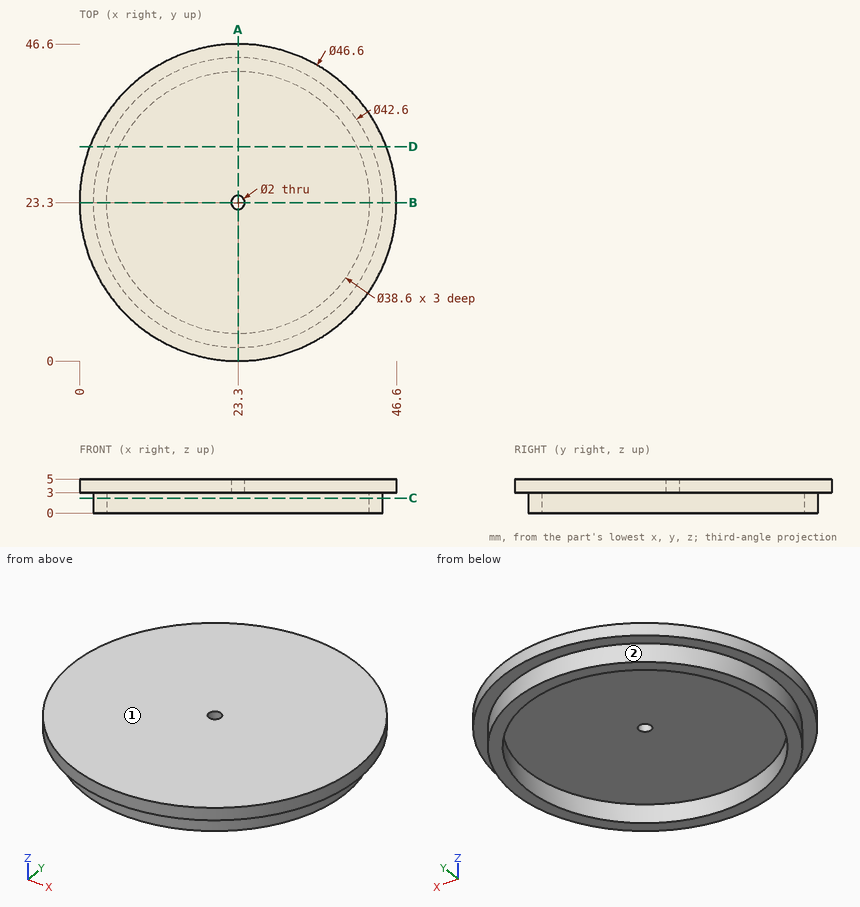
Print and shaded views of the part. All mm, measured from the part's lowest x, y and z. A direction names the side the tool comes from. Coordinates: 2 decimals unless noted, no trailing zeros. Order: outer loops, then holes, each group sorted by start corner. A loop starts at its lowest first (then second) coordinate and runs counter-clockwise, first axis right, second up. Notation, with made-up numbers: (49, -12) -> (64, -12) arc R11 cw to (64, -8) -> close; hole circle Ø6 at (30.25, 66). An arc over 180 degrees is marked (long way). Use one line per item in the form item = value. Start each with the question number.
1) Band-saw the part on C-C on z = 2.2. Give the cut face in (x, y), then the cut area to 3 significant figures.
2) Drill centre lines: L1, parallel to Y at x = 23, z = 2.5; L2, parallel to Y at x = 23.3, z = 3.4; L3, parallel to Z at x = 32, y = 44. Where is each one in solid material? Low to high. Write a range as [from, to].
3) Band-saw the part on D-D on y = 31.5. Give the cut face in (x, z).
4) Band-saw the part on A-A on x = 23.3. Give the cut face in (y, z).
5) Tool access for the marked faces 1 and 2: list every direction of +Z, -Z, +X, -X, +Y, -Y with a clear straight run to the whole face (end or side of a thin tool).
6) Drop flat-ended pins along their axis: pin 1 (3 mm diameter, centred on y = 10, z = 3, fed in from -X); pin 2 (3 mm diameter, centred on y = 16.5, z = 2, fed in from +X); pin 3 (1.5 mm diameter, centred on y = 31, z = 1, fed in from +X); pin 4 (1.2 mm diameter, centred on x = 23.3, y = 23.3, fed in from +Z). Give the stop position or say it passes through.
Entries:
q1.outline = circle Ø42.6 at (23.3, 23.3); hole circle Ø38.6 at (23.3, 23.3)
q1.area = 255 mm2
q2.L1 = [2, 4], [42.6, 44.6]
q2.L2 = [0, 22.3], [24.3, 46.6]
q2.L3 = [3, 5]
q3.outline = (1.49, 3) -> (3.64, 3) -> (3.64, 0) -> (5.83, 0) -> (5.83, 3) -> (40.77, 3) -> (40.77, 0) -> (42.96, 0) -> (42.96, 3) -> (45.11, 3) -> (45.11, 5) -> (1.49, 5) -> close
q4.outline = (0, 3) -> (2, 3) -> (2, 0) -> (4, 0) -> (4, 3) -> (22.3, 3) -> (22.3, 5) -> (0, 5) -> close; (24.3, 3) -> (42.6, 3) -> (42.6, 0) -> (44.6, 0) -> (44.6, 3) -> (46.6, 3) -> (46.6, 5) -> (24.3, 5) -> close
q5.face_1 = +Z, +X, -X, +Y, -Y
q5.face_2 = -Z
q6.pin_1 = 3.21
q6.pin_2 = 45.9
q6.pin_3 = 43.43
q6.pin_4 = through
